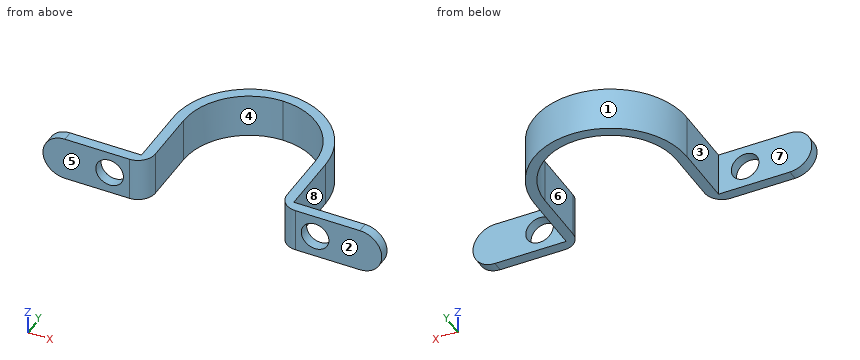
from build123d import *

# Parameters (mm, degrees)
BOSS_EXTRUDE1_DEPTH = 12.7
FILLET1_R           = 19.05
FILLET4_RADIUS      = 22.05
FILLET4_LENGTH      = 12.7
SKETCH2_R           = 4
CUT_EXTRUDE1_DEPTH  = 68.509113983
FILLET5_RADIUS      = 6.35
FILLET5_LENGTH      = 3
FILLET6_RADIUS      = 6.35
FILLET6_LENGTH      = 3
FILLET7_R           = 5


with BuildPart() as part:
    # Sketch1 → Boss-Extrude1 (new body)
    with BuildSketch(Plane.XY):
        Polygon((-45.220982698, 0), (-18.220982698, 0), (-18.220982698, 40), (25.879017302, 40), (25.879017302, 0), (52.879017302, 0), (52.879017302, -3), (22.879017302, -3), (22.879017302, 37), (-15.220982698, 37), (-15.220982698, -3), (-45.220982698, -3), align=None)
    extrude(amount=BOSS_EXTRUDE1_DEPTH)

    # Fillet1
    fillet1_edges = [part.edges().sort_by_distance(p)[0] for p in [
        (22.879017302, 37, 6.35),
        (-15.220982698, 37, 6.35),
    ]]
    fillet(fillet1_edges, radius=FILLET1_R - 0.0001)  # a hair under: the kernel refuses the full size

    # Fillet4: full round fillet: the end face becomes a half cylinder, R = half its width
    fillet4_face = Plane((3.829017302, 40, 6.35), x_dir=(0, 0, 1), z_dir=(0, 1, 0))  # on the end face: x along it, z out of the body
    fillet4_slab = fillet4_face.offset(-FILLET4_RADIUS / 2) * Box(FILLET4_LENGTH, 2 * FILLET4_RADIUS, FILLET4_RADIUS, mode=Mode.PRIVATE)  # the body's end, R deep
    fillet4_round = Plane((3.829017302, 17.95, 6.35), x_dir=(0, 1, 0), z_dir=(0, 0, 1)) * Cylinder(FILLET4_RADIUS, FILLET4_LENGTH, mode=Mode.PRIVATE)  # its axis R under the face
    add(fillet4_slab - fillet4_round, mode=Mode.SUBTRACT)

    # Sketch2 → Cut-Extrude1 (cut, through all)
    with BuildSketch(Plane(origin=(0, 0, 0), x_dir=(1, 0, 0), z_dir=(0, 1, 0))):
        with Locations(Location((-25.920982698, -6.35, 0), (0, 0, 270))):
            Circle(SKETCH2_R)
        with Locations(Location((33.579017302, -6.35, 0), (0, 0, 270))):
            Circle(SKETCH2_R)
    extrude(amount=-CUT_EXTRUDE1_DEPTH, mode=Mode.SUBTRACT)

    # Fillet5: full round fillet: the end face becomes a half cylinder, R = half its width
    fillet5_face = Plane((-45.220982698, -1.5, 6.35), x_dir=(0, -1, 0), z_dir=(-1, 0, 0))  # on the end face: x along it, z out of the body
    fillet5_slab = fillet5_face.offset(-FILLET5_RADIUS / 2) * Box(FILLET5_LENGTH, 2 * FILLET5_RADIUS, FILLET5_RADIUS, mode=Mode.PRIVATE)  # the body's end, R deep
    fillet5_round = Plane((-38.870982698, -1.5, 6.35), x_dir=(-1, 0, 0), z_dir=(0, -1, 0)) * Cylinder(FILLET5_RADIUS, FILLET5_LENGTH, mode=Mode.PRIVATE)  # its axis R under the face
    add(fillet5_slab - fillet5_round, mode=Mode.SUBTRACT)

    # Fillet6: full round fillet: the end face becomes a half cylinder, R = half its width
    fillet6_face = Plane((52.879017302, -1.5, 6.35), x_dir=(0, 1, 0), z_dir=(1, 0, 0))  # on the end face: x along it, z out of the body
    fillet6_slab = fillet6_face.offset(-FILLET6_RADIUS / 2) * Box(FILLET6_LENGTH, 2 * FILLET6_RADIUS, FILLET6_RADIUS, mode=Mode.PRIVATE)  # the body's end, R deep
    fillet6_round = Plane((46.529017302, -1.5, 6.35), x_dir=(1, 0, 0), z_dir=(0, 1, 0)) * Cylinder(FILLET6_RADIUS, FILLET6_LENGTH, mode=Mode.PRIVATE)  # its axis R under the face
    add(fillet6_slab - fillet6_round, mode=Mode.SUBTRACT)

    # Fillet7
    fillet7_edges = [part.edges().sort_by_distance(p)[0] for p in [
        (22.879017302, -3, 6.35),
        (-15.220982698, -3, 6.35),
    ]]
    fillet(fillet7_edges, radius=FILLET7_R)


solid = part.part
Verification items for the finished model (mm, model axes). Face numbers are marked on the shaded views. A direction names the side the tool comes from. Coordinates: 2 decimals unless noted, no trailing zeros. Loops run counter-clockwise (first coordinate to the right, second up) from the corner with the lowest first, then second, coordinate; pieces in that order, holes last. Notation, with made-up numbers: (44, 23.5) -> (94, 23.5) arc R19 cw to (94, 50.5) -> close; hole circle Ø8 at (41.25, -6.5). An arc over 180 degrees is marked (long way). Write each question's results on one line, items separated by ' | '.
Item 1: Section check A-A, the plane y = 9. Enter the section's corners in (x, z).
Found:
outline: (-18.22, 0) -> (-15.22, 0) -> (-15.22, 12.7) -> (-18.22, 12.7) -> close; (22.88, 0) -> (25.88, 0) -> (25.88, 12.7) -> (22.88, 12.7) -> close
Item 2: Section check C-C, the plane x = -27. Enter the section's corners in (y, z).
Found:
outline: (-3, 0) -> (0, 0) -> (0, 2.5) -> (-3, 2.5) -> close; (-3, 10.2) -> (0, 10.2) -> (0, 12.7) -> (-3, 12.7) -> close
Item 3: Gauge pin test, flat ends, axial feed: pin 1 (3 mm diameter, centred on y = 4, z = 6.5, fed in from -X); pin 2 (4 mm diameter, centred on x = 19.5, z = 6, fed in from +Y); pin 3 (4 mm diameter, centred on y = 7.5, z = 6, fed in from +X); pin 4 (7 mm diameter, centred on x = -25.92, z = 6.35, fed in from -Y). Record the tip position at first contact, or that the pin passes through.
Found:
pin 1: stops at x = -18.22 | pin 2: stops at y = 35.25 | pin 3: stops at x = 25.88 | pin 4: passes through
Item 4: Tool access check on the marked faces 5, 6, 7 and 8. Record the directions out of +Z, -Z, +X, -X, +Y, -Y that give a thin tool (end or side, any length) a straight path to the whole face; none if there is none.
Found:
face 5: +Z, -Z, +X, -X, -Y | face 6: +Z, -Z, -Y | face 7: +Z, -Z, -X, +Y | face 8: +Z, -Z, +X, +Y
Item 5: Section check B-B, the plane z = 6.35. Count the separate pieces of the cut face and the enclosed holes in it, plus the area to 3 significant figures.
Found:
separate pieces: 3 | enclosed holes: 0 | area: 423 mm2
Item 6: Material ranges on L1, parallel to X at y = -1.15, z = 6.35; L2, parallel to X at y = 6.5, z = 7; L3, parallel to X at y = -1.8, z = 6.35, recorded low to high.
Found:
L1: x = -45.22 to -29.92, -21.92 to -16.34, 24 to 29.58, 37.58 to 52.88 | L2: x = -18.22 to -15.22, 22.88 to 25.88 | L3: x = -45.22 to -29.92, -21.92 to -16.97, 24.63 to 29.58, 37.58 to 52.88
Item 7: Section check D-D, the plane x = -17. Enter the section's corners in (y, z).
Found:
outline: (-1.82, 0) -> (25.19, 0) -> (25.19, 12.7) -> (-1.82, 12.7) -> close
Item 8: Mould release check, pull along X, two halves, no side actions. Record for the marked faces 1, 2, 3 and 4: +X half, -X half, draft (parallel to the pull), parting line (faces both ways), or undercut.
Found:
face 1: parting line | face 2: draft | face 3: -X half | face 4: undercut
